```python
from build123d import *

# Parameters (mm, degrees)
F0_W     = 273.05
F0_H     = 114.3
F1_DEPTH = 19.05
F3_DEPTH = 25.4
F4_DEPTH = 25.4
F5_R     = 6.35
F6_R     = 6.35


with BuildPart() as f1:
    # F0 (on Front) → F1 (new body)
    with BuildSketch(Plane.XZ):
        with Locations((136.525, 57.15)):
            Rectangle(F0_W, F0_H)
    extrude(amount=F1_DEPTH)

    # F2 (on face) → F3 (cut)
    with BuildSketch(Plane.XZ.offset(19.05)):
        with BuildLine():
            ThreePointArc((72.8078575524, 38.1187458841), (75.3373142564, 44.2364484398), (76.2, 50.8))
            ThreePointArc((76.2, 50.8), (32.4977854296, 68.4121816315), (51.7756738724, 25.4187458841))
            Line((51.7756738724, 25.4187458841), (64.3298327923, 38.1187458841))
            Line((64.3298327923, 38.1187458841), (72.8078575524, 38.1187458841))
        make_face()
        with BuildLine():
            ThreePointArc((200.2421424476, 38.1187458841), (209.1205225089, 29.0565683295), (221.2743261276, 25.4187458841))
            Line((221.2743261276, 25.4187458841), (223.2256738724, 25.4187458841))
            Line((223.2256738724, 25.4187458841), (207.7043950558, 38.1187458841))
            Line((207.7043950558, 38.1187458841), (200.2421424476, 38.1187458841))
        make_face()
        with BuildLine():
            Line((223.2256738724, 25.4187458841), (221.2743261276, 25.4187458841))
            ThreePointArc((221.2743261276, 25.4187458841), (222.25, 25.4), (223.2256738724, 25.4187458841))
        make_face()
        with BuildLine():
            Line((64.3298327923, 38.1187458841), (51.7756738724, 25.4187458841))
            ThreePointArc((51.7756738724, 25.4187458841), (63.9294774911, 29.0565683295), (72.8078575524, 38.1187458841))
            Line((72.8078575524, 38.1187458841), (64.3298327923, 38.1187458841))
        make_face()
        with BuildLine():
            ThreePointArc((247.65, 50.8), (215.6864484398, 75.3373142564), (200.2421424476, 38.1187458841))
            Line((200.2421424476, 38.1187458841), (207.7043950558, 38.1187458841))
            Line((207.7043950558, 38.1187458841), (223.2256738724, 25.4187458841))
            ThreePointArc((223.2256738724, 25.4187458841), (240.5522145704, 33.1878183685), (247.65, 50.8))
        make_face()
        with BuildLine():
            Line((100.33, 57.15), (151.0539650917, 57.15))
            Line((151.0539650917, 57.15), (172.72, 57.15))
            ThreePointArc((172.72, 57.15), (180.802230509, 60.497769491), (184.15, 68.58))
            Line((184.15, 68.58), (184.15, 114.3))
            Line((184.15, 114.3), (88.9, 114.3))
            Line((88.9, 114.3), (88.9, 68.58))
            ThreePointArc((88.9, 68.58), (92.247769491, 60.497769491), (100.33, 57.15))
        make_face()
    extrude(amount=-F3_DEPTH, mode=Mode.SUBTRACT)

    # F2 (on face) → F4 (cut)
    with BuildSketch(Plane.XZ.offset(19.05)):
        with BuildLine():
            ThreePointArc((72.8078575524, 38.1187458841), (75.3373142564, 44.2364484398), (76.2, 50.8))
            ThreePointArc((76.2, 50.8), (32.4977854296, 68.4121816315), (51.7756738724, 25.4187458841))
            Line((51.7756738724, 25.4187458841), (64.3298327923, 38.1187458841))
            Line((64.3298327923, 38.1187458841), (72.8078575524, 38.1187458841))
        make_face()
        with BuildLine():
            ThreePointArc((200.2421424476, 38.1187458841), (209.1205225089, 29.0565683295), (221.2743261276, 25.4187458841))
            Line((221.2743261276, 25.4187458841), (223.2256738724, 25.4187458841))
            Line((223.2256738724, 25.4187458841), (207.7043950558, 38.1187458841))
            Line((207.7043950558, 38.1187458841), (200.2421424476, 38.1187458841))
        make_face()
        with BuildLine():
            Line((223.2256738724, 25.4187458841), (221.2743261276, 25.4187458841))
            ThreePointArc((221.2743261276, 25.4187458841), (222.25, 25.4), (223.2256738724, 25.4187458841))
        make_face()
        with BuildLine():
            Line((64.3298327923, 38.1187458841), (51.7756738724, 25.4187458841))
            ThreePointArc((51.7756738724, 25.4187458841), (63.9294774911, 29.0565683295), (72.8078575524, 38.1187458841))
            Line((72.8078575524, 38.1187458841), (64.3298327923, 38.1187458841))
        make_face()
        with BuildLine():
            ThreePointArc((247.65, 50.8), (215.6864484398, 75.3373142564), (200.2421424476, 38.1187458841))
            Line((200.2421424476, 38.1187458841), (207.7043950558, 38.1187458841))
            Line((207.7043950558, 38.1187458841), (223.2256738724, 25.4187458841))
            ThreePointArc((223.2256738724, 25.4187458841), (240.5522145704, 33.1878183685), (247.65, 50.8))
        make_face()
    extrude(amount=-F4_DEPTH, mode=Mode.SUBTRACT)

    # F5
    f5_edges = [f1.edges().sort_by_distance(p)[0] for p in [
        (44.45, -19.05, 114.3),
    ]]
    fillet(f5_edges, radius=F5_R)

    # F6
    f6_edges = [f1.edges().sort_by_distance(p)[0] for p in [
        (228.6, -19.05, 114.3),
    ]]
    fillet(f6_edges, radius=F6_R)


solid = f1.part
```
Geometry check sheet. Reference: the model listing, model coordinates, mm. A direction names the side the tool comes from. Round coordinates to 2 decimals unless told otherwise and drop trailing zeros. Order: outer loops, then holes, each group sorted by start corner. A loop starts at its lowest first (then second) coordinate and runs counter-clockwise, first axis right, second up. Notation, with made-up numbers: (8.5, 46) - (63.5, 46) arc R34 cw to (63.5, 77) - close; hole circle Ø9 at (85, 7.5). An arc over 180 degrees is marked (long way). Use a Markdown table: item, result. Add a question column.
(1) Release check for a two-part mould opening along X. For faces 3 (the cylindrical face through (180.713, -9.658, 60.409)), 4 (the flat face through (273.05, -9, 56)), 5 (the cylindrical face through (45.07, -17.14, 112.49)) record: pulls with the +X half, pulls with the -X half, needs draft (parallel to the pull), parting line crosses it, or undercut.
(2) Sectioned sample at B-B, the plane x = 203. Enter the section's corners in (y, z).
(3) Material ranges on line 1 along Z through (x, y) = (51.5, -13.5); line 2 along Z through (x, y) = (222.25, -8.25); line 3 along X through (y, z) = (-14.5, 50.8), recorded low to high. Write a range as [from, to].
(4) Sectioned sample at C-C, the plane y = -5.25. Enter the section's corners in (x, z).
(5) Sectioned sample at A-A, the plane z = 90.5. Enter the section's corners in (x, y).
(6) Tool access check on faces 1 (the flat face through (0, -9, 56)), 2 (the cylindrical face through (92.159, -9.658, 60.587)). Record the directions out of +Z, -Z, +X, -X, +Y, -Y that give a thin tool (end or side, any length) a straight path to the whole face; none if there is none.
(7) Sectioned sample at D-D, the plane z = 63. Enter the section's corners in (x, y).
(8) Depth check by flat-ended pin: pin 1 (1 mm diameter, centred on x = 158.5, y = -5.5, fed in from +Z); pin 2 (10 mm diameter, centred on x = 97, y = -13.5, fed in from +Z). Enter the tip coordinate at first touch or a pass-through.
Answers below:
| question | item | result |
|---|---|---|
| 1 | face 3 | undercut |
| 1 | face 4 | pulls with the +X half |
| 1 | face 5 | needs draft |
| 2 | outline | (-19.05, 0) - (0, 0) - (0, 34.23) - (-19.05, 34.23) - close; (-19.05, 67.37) - (0, 67.37) - (0, 114.3) - (-12.7, 114.3) arc R6.35 ccw to (-19.05, 107.95) - close |
| 3 | line 1 | [0, 25.41], [76.19, 114.25] |
| 3 | line 2 | [0, 25.4], [76.2, 114.3] |
| 3 | line 3 | [0, 25.4], [76.2, 196.85], [247.65, 273.05] |
| 4 | outline | (0, 0) - (273.05, 0) - (273.05, 114.3) - (184.15, 114.3) - (184.15, 68.58) arc R11.43 cw to (172.72, 57.15) - (100.33, 57.15) arc R11.43 cw to (88.9, 68.58) - (88.9, 114.3) - (0, 114.3) - close; hole circle Ø50.8 at (50.8, 50.8); hole circle Ø50.8 at (222.25, 50.8) |
| 5 | outline | (0, -19.05) - (88.9, -19.05) - (88.9, 0) - (0, 0) - close; (184.15, -19.05) - (273.05, -19.05) - (273.05, 0) - (184.15, 0) - close |
| 6 | face 1 | +Z, -Z, -X, +Y, -Y |
| 6 | face 2 | +Z, +Y, -Y |
| 7 | outline | (0, -19.05) - (28.52, -19.05) - (28.52, 0) - (0, 0) - close; (73.08, -19.05) - (90.35, -19.05) - (90.35, 0) - (73.08, 0) - close; (182.7, -19.05) - (199.97, -19.05) - (199.97, 0) - (182.7, 0) - close; (244.53, -19.05) - (273.05, -19.05) - (273.05, 0) - (244.53, 0) - close |
| 8 | pin 1 | z = 57.15 |
| 8 | pin 2 | z = 60.75 |
